The listing builds one solid part. Answer for the finished solid, in the listing's coordinates (mm). Give positions to 0.01 mm unless a question says otherwise; leave off trailing zeros.
Autodesk Inventor part; units mm, degrees
ref_plane "YZ Plane" through (0, 0, 0) normal (1, 0, 0) x (0, 1, 0)
ref_plane "XZ Plane" through (0, 0, 0) normal (0, 1, 0) x (-1, 0, 0)
ref_plane "XY Plane" through (0, 0, 0) normal (0, 0, 1) x (1, 0, 0)
sketch "Sketch1" plane through (0, 0, 0) normal (0, 1, 0) x (-1, 0, 0)
  circle A0 centre (0, 0) radius 19.05
  arc A1 (4.4642, 39.1161) -> (-1.9997, -39.3192) centre (0, 0) ccw
  line L0 (-1.9997, -39.3192) -> (49.0185, -41.9138) construction
  line L1 (263.1315, -247.3812) -> (302.3964, -370.4331) construction
  spline S0 degree 4 poles (-1.9997, -39.3192) (49.0185, -41.9138) (105.6374, -72.1982) (173.8913, -120.1961) (263.1315, -247.3812) (302.3964, -370.4331) knots 1 1 1 1 1 1.581444 2 2 2 2 2
  line L2 (4.4642, 39.1161) -> (78.1887, 30.7022) construction
  line L3 (339.9032, -237.0622) -> (377.1456, -345.6975) construction
  spline S1 degree 4 poles (4.4642, 39.1161) (78.1887, 30.7022) (179.8099, -32.9721) (261.2925, -118.1743) (339.9032, -237.0622) (377.1456, -345.6975) knots 0 0 0 0 0 1 2 2 2 2 2
  circle A2 centre (339.9032, -358.4649) radius 19.05
  arc A3 (302.3964, -370.4331) -> (377.1456, -345.6975) centre (339.9032, -358.4649) ccw
  circle A4 centre (339.9032, -358.4649) radius 15.8726 construction
  arc A5 (265.0359, -199.854) -> (201.2966, -118.1743) centre (2.3813, -339.1088) ccw construction
  arc A6 (280.7447, -191.5256) -> (213.1932, -104.9608) centre (2.3813, -339.1088) ccw
  arc A7 (249.3272, -208.1825) -> (189.3999, -131.3879) centre (2.3813, -339.1088) ccw
  arc A8 (249.3272, -208.1825) -> (280.7447, -191.5256) centre (265.0359, -199.854) ccw
  arc A9 (213.1932, -104.9608) -> (189.3999, -131.3879) centre (201.2966, -118.1743) ccw
  arc A10 (161.0182, -77.5529) -> (62.8262, -16.2966) centre (-36.5592, -284.9364) ccw construction
  arc A11 (173.2826, -64.6798) -> (68.9954, 0.3788) centre (-36.5592, -284.9364) ccw
  arc A12 (148.7539, -90.4259) -> (56.657, -32.9721) centre (-36.5592, -284.9364) ccw
  arc A13 (148.7539, -90.4259) -> (173.2826, -64.6798) centre (161.0182, -77.5529) ccw
  arc A14 (68.9954, 0.3788) -> (56.657, -32.9721) centre (62.8262, -16.2966) ccw
  line L4 (78.1887, 30.7022) -> (179.8099, -32.9721) construction
  line L5 (179.8099, -32.9721) -> (261.2925, -118.1743) construction
  line L6 (261.2925, -118.1743) -> (339.9032, -237.0622) construction
  line L7 (49.0185, -41.9138) -> (105.6374, -72.1982) construction
  line L8 (105.6374, -72.1982) -> (173.8913, -120.1961) construction
  line L9 (173.8913, -120.1961) -> (263.1315, -247.3812) construction
  dimension "d0" = 38.1
  dimension "d1" = 20.32
  dimension "d2" = 38.1
  dimension "d3" = 20.32
  dimension "d6" = 17.78
  dimension "d7" = 17.78
extrude "Extrusion1" add sketch "Sketch1" along normal blind 20
equation "\"d1\" = d3"
equation "\"d2\" = d0"
equation "\"d7\" = d6"
properties part number "Profile" material "Aluminum 6061"
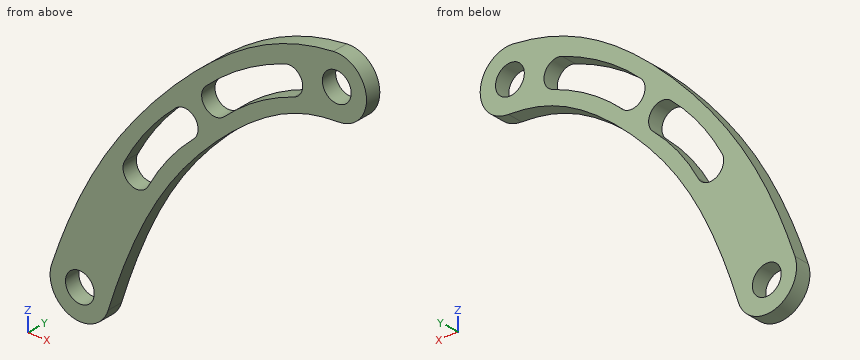
1) Given P1, Ø8, axis at x = -152, y = 15.5, coming from the +Z side; P2, Ø10, axis at y = 10, z = -76.5, coming from the +X side; P3, Ø5, axis at y = 16, z = -262, coming from the +X side, each flat-ended and moving along its own axis, determine where each tip first touches the part or whether it passes through.
Geometry says:
P1: stops at z = -20.59
P2: stops at x = -95.56
P3: stops at x = -258.79
2) Straight lines are drawn through the part: probe 1 along X at (y, z) = (16.75, 15.5); probe 2 along X at (y, z) = (9.5, -104); probe 3 along X at (y, z) = (5, -7). For each, find the intervals that lie inside material, in ascending order.
Geometry says:
probe 1: x = -88.26 to -11.07, 11.07 to 36.19
probe 2: x = -237.79 to -212.03, -190.56 to -138.83
probe 3: x = -128.52 to -87.13, -47.67 to -17.72, 17.72 to 38.74
3) Find section A-A (y = 9.5). Count the separate pieces of the cut face and the enclosed holes in it, then the cut area to 3 significant figures.
Geometry says:
separate pieces: 1
enclosed holes: 4
area: 30,900 mm2
